Geometry check sheet. Reference: the model listing, model coordinates, mm. A direction names the side the tool comes from. Give positions to 0.01 mm unless a question says otherwise; leave off trailing zeros. Loops run counter-clockwise (first coordinate to the right, second up) from the corner with the lowest first, then second, coordinate; pieces in that order, holes last. Notation, with made-up numbers: (76.5, 71) -> (112.5, 71) arc R11 ccw to (112.5, 79) -> close; hole circle Ø9 at (-9, 52.5). An arc over 180 degrees is marked (long way). Answer as a JSON object with one key per item and string values.
from build123d import *

# Parameters (mm, degrees)
SKETCH_1_R          = 5
SKETCH_1_R_2        = 8
EXTRUDE_1_DEPTH     = 35
SKETCH_2_R          = 8
SKETCH_2_R_2        = 6
EXTRUDE_2_DEPTH     = 82.5
SKETCH_3_W          = 42.302016602
SKETCH_3_H          = 114.861822868
CUT_EXTRUDE_1_DEPTH = 25.5
SKETCH_4_W          = 64.639494707
SKETCH_4_H          = 157.942491396
CUT_EXTRUDE_2_DEPTH = 31
SKETCH_5_R          = 36.84087404
SKETCH_5_R_2        = 7.5
EXTRUDE_3_DEPTH     = 128.2
CUT_EXTRUDE_3_DEPTH = 64


with BuildPart() as part:
    # Эскиз1 → Бобышка-Вытянуть1 (new, symmetric)
    with BuildSketch(Plane.XY):
        with BuildLine():
            Line((46.485752599, 163.525957525), (-16.969355429, 234.506193035))
            Line((-16.969355429, 234.506193035), (139.491938283, 374.379894827))
            Line((139.491938283, 374.379894827), (-27.598469683, 354.342788957))
            Line((-27.598469683, 354.342788957), (-509.881731069, 581.127761724))
            Line((-509.881731069, 581.127761724), (-518.721104493, 585.424916142))
            Line((-518.721104493, 585.424916142), (-574.35237116, 470.989759218))
            Line((-574.35237116, 470.989759218), (-563.968249487, 466.106813988))
            Line((-563.968249487, 466.106813988), (-554.670789116, 461.734851563))
            ThreePointArc((-554.670789116, 461.734851563), (-526.024716524, 439.039773197), (-510.461622358, 405.972354837))
            Line((-510.461622358, 405.972354837), (-426.739911846, 12.092674745))
            ThreePointArc((-426.739911846, 12.092674745), (-398.833735071, -33.446066906), (-348.488103787, -51.27438999))
            Line((-348.488103787, -51.27438999), (-48.06941217, -51.27438999))
            ThreePointArc((-48.06941217, -51.27438999), (-31.671926194, -46.396540648), (-20.606737964, -33.349220236))
            Line((-20.606737964, -33.349220236), (-0.352735385, 12.715946965))
            ThreePointArc((-0.352735385, 12.715946965), (0.577617407, 17.143384722), (-0.352735385, 21.570822479))
            Line((-0.352735385, 21.570822479), (-24.532087898, 76.563701639))
            Line((-24.532087898, 76.563701639), (45.102587172, 138.81590181))
            ThreePointArc((45.102587172, 138.81590181), (50.911789988, 150.884466728), (46.485752599, 163.525957525))
        make_face()
        with Locations((33.439142029, 151.862512381)):
            Circle(SKETCH_1_R, mode=Mode.SUBTRACT)
        with Locations((-10.422382593, 17.143384722)):
            Circle(SKETCH_1_R_2, mode=Mode.SUBTRACT)
        Polygon((1.669070396, 153.64086793), (-49.881296122, 211.304581219), (-49.881296122, 107.555728133), align=None, mode=Mode.SUBTRACT)
        with BuildLine():
            Line((-424.341826107, 331.410461473), (-130.558293442, 283.519373673))
            Line((-130.558293442, 283.519373673), (-114.7080306, 280.935544953))
            ThreePointArc((-114.7080306, 280.935544953), (-90.449389812, 287.688615998), (-79.881296122, 310.544709653))
            Line((-79.881296122, 310.544709653), (-79.881296122, 326.732272667))
            ThreePointArc((-79.881296122, 326.732272667), (-84.553646066, 342.810523277), (-97.115305634, 353.880559664))
            Line((-97.115305634, 353.880559664), (-106.521117185, 358.30347227))
            Line((-106.521117185, 358.30347227), (-405.741591683, 499.006483537))
            ThreePointArc((-405.741591683, 499.006483537), (-434.47055763, 497.258657451), (-448.506342859, 472.130881716))
            Line((-448.506342859, 472.130881716), (-449.513852316, 361.29231135))
            ThreePointArc((-449.513852316, 361.29231135), (-442.459263359, 341.691796922), (-424.341826107, 331.410461473))
        make_face(mode=Mode.SUBTRACT)
        with BuildLine():
            Line((-438.961647095, 261.980792175), (-387.614007817, 20.409142377))
            ThreePointArc((-387.614007817, 20.409142377), (-373.660919429, -2.360228448), (-348.488103787, -11.27438999))
            Line((-348.488103787, -11.27438999), (-109.881296122, -11.27438999))
            ThreePointArc((-109.881296122, -11.27438999), (-88.668092686, -2.487593425), (-79.881296122, 18.72561001))
            Line((-79.881296122, 18.72561001), (-79.881296122, 219.356726902))
            ThreePointArc((-79.881296122, 219.356726902), (-87.025202466, 238.788633212), (-105.054561643, 248.965891603))
            Line((-105.054561643, 248.965891603), (-404.790484594, 297.8273076))
            ThreePointArc((-404.790484594, 297.8273076), (-431.331787712, 288.917841178), (-438.961647095, 261.980792175))
        make_face(mode=Mode.SUBTRACT)
    extrude(amount=EXTRUDE_1_DEPTH, both=True)

    # Эскиз2 → Бобышка-Вытянуть2 (add, symmetric)
    with BuildSketch(Plane.XY):
        with Locations((-10.422382593, 17.143384722)):
            Circle(SKETCH_2_R)
        with Locations((-10.422382593, 17.143384722)):
            Circle(SKETCH_2_R_2, mode=Mode.SUBTRACT)
    extrude(amount=EXTRUDE_2_DEPTH, both=True)

    # Эскиз3 → Вырез-Вытянуть1 (cut, symmetric)
    with BuildSketch(Plane.XY):
        with Locations((35.909206886, 152.283379398)):
            Rectangle(SKETCH_3_W, SKETCH_3_H)
    extrude(amount=CUT_EXTRUDE_1_DEPTH, both=True, mode=Mode.SUBTRACT)

    # Эскиз4 → Вырез-Вытянуть2 (cut, symmetric)
    with BuildSketch(Plane.XY):
        with Locations((-17.561548768, 155.534947337)):
            Rectangle(SKETCH_4_W, SKETCH_4_H)
    extrude(amount=CUT_EXTRUDE_2_DEPTH, both=True, mode=Mode.SUBTRACT)

    # Эскиз5 → Бобышка-Вытянуть3 (add)
    with BuildSketch(Plane(origin=(131.039320596, 269.551748755, 0), x_dir=(0.8993583813402204, -0.4372121932347024, 0), z_dir=(0.4372121932347024, 0.8993583813402204, 0))):
        with Locations(Location((-733.971084464, 0, 0), (0, 0, 180))):
            Circle(SKETCH_5_R)
        with Locations(Location((-733.971084464, 0, 0), (0, 0, 180))):
            Circle(SKETCH_5_R_2, mode=Mode.SUBTRACT)
    extrude(amount=-EXTRUDE_3_DEPTH)

    # Эскиз6 → Вырез-Вытянуть3 (cut, symmetric)
    with BuildSketch(Plane.XY):
        Polygon((-612.900055289, 502.26219729), (-540.3281869, 466.982261723), (-526.024716524, 439.039773197), (-623.276117578, 486.317364902), (-615.524730273, 502.26219729), align=None)
    extrude(amount=CUT_EXTRUDE_3_DEPTH, both=True, mode=Mode.SUBTRACT)


solid = part.part
1) Section check D-D on z = 63.5. Record the cut outline in (x, y).
Geometry check:
{"outline": "circle Ø16 at (-10.42, 17.14); hole circle Ø12 at (-10.42, 17.14)"}
2) Section check B-B on x = -217. Record the cut outline in (y, z).
Geometry check:
{"outline": "(-51.27, -35) -> (-11.27, -35) -> (-11.27, 35) -> (-51.27, 35) -> close; (267.21, -35) -> (297.61, -35) -> (297.61, 35) -> (267.21, 35) -> close; (410.25, -35) -> (443.41, -35) -> (443.41, 35) -> (410.25, 35) -> close"}
3) Tool access check on faces 1 (the face through (-34, 234.506, 0)), 2 (the face through (-79.881, 118, 0)), 3 (the face through (-6.731, 10.046, 59.082)), 4 (the face through (-569.06, 480.95, 0.52)). Record the directions out of +Z, -Z, +X, -X, +Y, -Y that give a thin tool (end or side, any length) a straight path to the whole face; none if there is none.
Geometry check:
{"face 1": "+X", "face 2": "+Z, -Z", "face 3": "+Z", "face 4": "+Z, -Z, -X, -Y"}
4) Depth check by flat-ended pin: P1, Ø11, axis at x = 34.5, y = 137.5, coming from the -Z side; P2, Ø7.5, axis at x = -42.5, z = -10.5, coming from the +Y side; P3, Ø11.5, axis at x = 33.44, y = 151.86, coming from the +Z side. Enter the tip coordinate at first touch or a pass-through.
Geometry check:
{"P1": "stops at z = -35", "P2": "stops at y = 363.11", "P3": "stops at z = 35"}
5) Section check A-A on y = 425. Record the cut outline in (x, z), plus the area to 3 significant figures.
Geometry check:
{"outline": "(-517.1, -35) -> (-448.93, -35) -> (-448.93, 35) -> (-517.1, 35) -> close; (-248.36, -35) -> (-177.86, -35) -> (-177.86, 35) -> (-248.36, 35) -> close", "area": "9,710 mm2"}
6) Draft check along Z on faces 5 (the face through (-7, 23, 82.5)), 6 (the face through (-533.28, 453.21, 0.49)), 7 (the face through (-11, 174, -31)), 8 (the face through (-11, 174, 31)). Enter one of: pulls with the +Z half, pulls with the -Z half, needs draft (parallel to the pull), parting line crosses it, or undercut.
Geometry check:
{"face 5": "pulls with the +Z half", "face 6": "needs draft", "face 7": "undercut", "face 8": "undercut"}
7) Section check C-C on y = 89. Record the cut outline in (x, z), plus the area to 3 significant figures.
Geometry check:
{"outline": "(-443.09, -35) -> (-402.19, -35) -> (-402.19, 35) -> (-443.09, 35) -> close; (-79.88, -35) -> (-10.62, -35) -> (-10.62, -31) -> (-49.88, -31) -> (-49.88, 31) -> (-10.62, 31) -> (-10.62, 35) -> (-79.88, 35) -> close", "area": "5,280 mm2"}
8) Material ranges on line 1 along Z through (x, y) = (13, 181); line 2 along X through (y, z) = (165, 15); line 3 along X through (y, z) = (65.5, -29), recorded low to high. Write a range as from..to.
Geometry check:
{"line 1": "z = -35..-31, 31..35", "line 2": "x = -459.24..-418.35, -79.88..-49.88", "line 3": "x = -438.09..-397.2, -79.88..-19.67"}
